Source: CAD feature listing. Evaluate the final solid. Frame: model axes, mm. Coordinates: 2 decimals unless noted, no trailing zeros. Write each loop counter-clockwise with the first axis right and the second up, starting at its lowest first coordinate (ties: lowest second). Pieces come first, ordered by that corner, then holes. Notation, with made-up numbers: (62, -6) - (79, -6) arc R33 cw to (79, 30) - close; hole circle Ø10 at (-36, 85). An arc over 180 degrees is marked (long way). One line per question, with ' | ' between items. Start each with the question number.
Q1. Cut plane A-A, the plane y = 0. Return loops of the section in (x, z) (3 decimals).
Q2. Cut plane D-D, the plane z = -0.6. Give the number of separate pieces and of enclosed holes in the cut face, plus the area to 3 significant figures.
Q3. Cut plane C-C, the plane z = -1.75. Return loops of the section in (x, y) (3 decimals), plus the area to 3 significant figures.
Q4. Line query: line 1 (X direction, y = -0.05, z = -2.6); line 2 (Z direction, x = 2, y = 0) (3 decimals); line 3 (Z direction, x = 0.25, y = 0). Output: solid intervals per line, ascending.
Q5. Cut plane B-B, the plane x = 0. Return loops of the section in (y, z), plus the area to 3 significant figures.
Q6. Contact query for flat-ended pins moving along their axis: P1, Ø0.5, axis at y = 0, z = 0, coming from the +X side; P2, Ø0.8, axis at y = 0, z = 0, coming from the -X side. Output: stop coordinate, or through.
```python
from build123d import *

# Parameters (mm, degrees)
F3_R = 0.275


with BuildPart() as f1:
    # F0 (on Top) → F1 (revolve)
    with BuildSketch(Plane.XY):
        with BuildLine():
            Line((0, 0), (0, 1))
            Line((0, 1), (-1, 1))
            ThreePointArc((-1, 1), (-1.3535533906, 0.8535533906), (-1.5, 0.5))
            Line((-1.5, 0.5), (-1.5, 0))
            Line((-1.5, 0), (0, 0))
        make_face()
    revolve(axis=Axis((-0.75, 0, 0), (-1, 0, 0)))

    # F2: F1 across face


with BuildPart() as f1_1:
    add(f1.part)
    add(f1.part.mirror(Plane.YZ))



with BuildPart() as f5:
    # F5: sweep along a path in F4
    with BuildLine(Plane.XZ) as f5_path:
        Line((0, 0), (3.645, 0))
        ThreePointArc((3.645, 0), (4.2106854249, -0.2343145751), (4.445, -0.8))
        Line((4.445, -0.8), (4.445, -4.5))
    # F3 (on Right) → F5 (sweep)
    with BuildSketch(Plane.YZ):
        Circle(F3_R)
    sweep(path=f5_path.line)


with BuildPart() as f1_2:
    add(f1_1.part)

    add(f5.part)  # F6 merges F5
    # F6: F5 across plane
    add(f5.part.mirror(Plane.YZ))


solid = f1_2.part
```
Reply:
1) outline: (-4.72, -4.5) - (-4.17, -4.5) - (-4.17, -0.8) arc R0.525 cw to (-3.645, -0.275) - (-1.5, -0.275) - (-1.5, -0.5) arc R0.5 ccw to (-1, -1) - (1, -1) arc R0.5 ccw to (1.5, -0.5) - (1.5, -0.275) - (3.645, -0.275) arc R0.525 cw to (4.17, -0.8) - (4.17, -4.5) - (4.72, -4.5) - (4.72, -0.8) arc R1.075 ccw to (3.645, 0.275) - (1.5, 0.275) - (1.5, 0.5) arc R0.5 ccw to (1, 1) - (-1, 1) arc R0.5 ccw to (-1.5, 0.5) - (-1.5, 0.275) - (-3.645, 0.275) arc R1.075 ccw to (-4.72, -0.8) - close
2) separate pieces: 3 | enclosed holes: 0 | area: 4.99 mm^2
3) outline: circle Ø0.55 at (-4.445, 0); circle Ø0.55 at (4.445, 0) | area: 0.475 mm^2
4) line 1: x = -4.72 to -4.17, 4.17 to 4.72 | line 2: z = -0.275 to 0.275 | line 3: z = -1 to 1
5) outline: circle Ø2 at (0, 0) | area: 3.14 mm^2
6) P1: stops at x = 4.57 | P2: stops at x = -4.64
